Geometry check sheet. Reference: the model listing, model coordinates, mm. Face numbers are marked on the shaded views. A direction names the side the tool comes from. Round coordinates to 2 decimals unless told otherwise and drop trailing zeros. Order: outer loops, then holes, each group sorted by start corner. A loop starts at its lowest first (then second) coordinate and runs counter-clockwise, first axis right, second up. Notation, with made-up numbers: M 62.25,11.25 L 103.25,11.25 A35 ccw 103.25,43.25 Z; hole C -30.75,44.25 d2. An arc over 180 degrees is marked long. Answer as a JSON object with one key per item and string values. Group by question number.
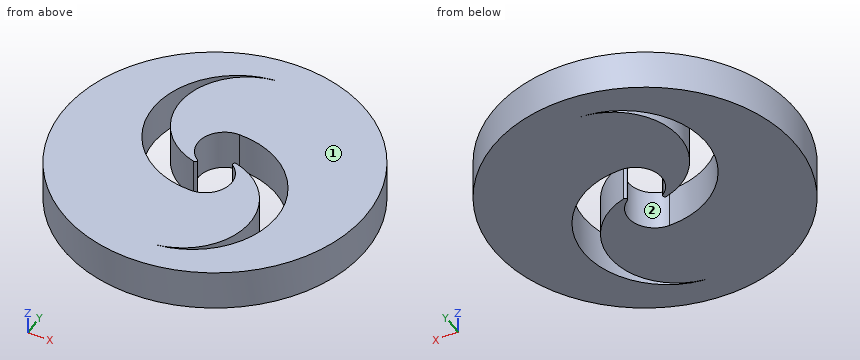
```python
from build123d import *

# Parameters (mm, degrees)
F0_R     = 22.5
F1_DEPTH = 6
F3_DEPTH = 25
F5_DEPTH = 25


with BuildPart() as f1:
    # F0 (on Top) → F1 (new body)
    with BuildSketch(Plane.XY):
        Circle(F0_R)
    extrude(amount=F1_DEPTH)

    # F2 (on face) → F3 (cut)
    with BuildSketch(Plane.XY.offset(6)):
        with BuildLine():
            ThreePointArc((0, 18.5), (-12.5, 6), (0, -6.5))
            ThreePointArc((0, -6.5), (2.5, -4), (0, -1.5))
            ThreePointArc((0, -1.5), (-10, 8.5), (0, 18.5))
        make_face()
        with BuildLine():
            ThreePointArc((0, 1.5), (10, -8.5), (0, -18.5))
            ThreePointArc((0, -18.5), (12.5, -6), (0, 6.5))
            ThreePointArc((0, 6.5), (-2.5, 4), (0, 1.5))
        make_face()
    extrude(amount=-F3_DEPTH, mode=Mode.SUBTRACT)

    # F4 (on face) → F5 (cut)
    with BuildSketch(Plane.XY.offset(6)):
        with BuildLine():
            ThreePointArc((2.298482, 0.635708), (2.202225, 1.007236), (2.550083, 1.169389))
            ThreePointArc((2.550083, 1.169389), (1.285713, 1.417003), (0, 1.5))
            Line((0, 1.5), (0, -1.5))
            ThreePointArc((0, -1.5), (-2.5, -4), (0, -6.5))
            ThreePointArc((0, -6.5), (3.748378, -3.769354), (2.298482, 0.635708))
        make_face()
        with BuildLine():
            Line((0, -1.5), (0, 1.5))
            ThreePointArc((0, 1.5), (2.5, 4), (0, 6.5))
            ThreePointArc((0, 6.5), (-3.748378, 3.769354), (-2.298482, -0.635708))
            ThreePointArc((-2.298482, -0.635708), (-2.202225, -1.007236), (-2.550083, -1.169389))
            ThreePointArc((-2.550083, -1.169389), (-1.285713, -1.417003), (0, -1.5))
        make_face()
    extrude(amount=-F5_DEPTH, mode=Mode.SUBTRACT)


solid = f1.part
```
1) Sectioned sample at C-C (z = 2.25). Record the boundary of the cut face in (x, y), then the cut area to 3 significant figures.
2) Thickness scan on line 1 along Y through (x, z) = (5, 1.95); line 2 along X through (y, z) = (5, 2.65); line 3 along X through (y, z) = (-3, 1.5). Record the ranges inside material, lowest first. Write a range as [from, to].
3) Sectioned sample at D-D (y = 5). Record the boundary of the cut face in (x, z).
4) Sectioned sample at A-A (y = -3). Record the boundary of the cut face in (x, z).
5) Sectioned sample at B-B (y = -8.5). Record the boundary of the cut face in (x, z).
6) Set-up check for the marked faces 1 and 2: record each of +Z, -Z, +X, -X, +Y, -Y from which the full face is reachable in a straight line by a thin tool's end or side.
Final values:
{
 "1": {"outline": "C 0,0 d45; hole M -2.55,-1.17 A10 cw 0,18.5 A12.5 ccw 0,-6.5 A3.94 ccw 2.3,0.64 A0.3 cw 2.55,1.17 A10 cw 0,-18.5 A12.5 ccw 0,6.5 A3.94 ccw -2.3,-0.64 A0.3 cw Z", "area": "1,360 mm^2"},
 "2": {"line 1": "y = [-21.94, -17.46], [-17.16, 0.16], [5.46, 21.94]", "line 2": "x = [-21.94, -12.46], [-9.37, -3.09], [5.94, 21.94]", "line 3": "x = [-22.3, -8.67], [3.91, 8.35], [12.13, 22.3]"},
 "3": {"outline": "M -21.94,0 L -12.46,0 L -12.46,6 L -21.94,6 Z; M -9.37,0 L -3.09,0 L -3.09,6 L -9.37,6 Z; M 5.94,0 L 21.94,0 L 21.94,6 L 5.94,6 Z"},
 "4": {"outline": "M -22.3,0 L -8.67,0 L -8.67,6 L -22.3,6 Z; M 3.91,0 L 8.35,0 L 8.35,6 L 3.91,6 Z; M 12.13,0 L 22.3,0 L 22.3,6 L 12.13,6 Z"},
 "5": {"outline": "M -20.83,0 L 10,0 L 10,6 L -20.83,6 Z; M 12.25,0 L 20.83,0 L 20.83,6 L 12.25,6 Z"},
 "6": {"face 1": "+Z, +X, -X, +Y, -Y", "face 2": "+Z, -Z"}
}
